Design review of the part built by this model. Coordinates are the model's own, in mm. Face numbers are marked on the shaded views. A direction names the side the tool comes from. Coordinates: 2 decimals unless noted, no trailing zeros. Loops run counter-clockwise (first coordinate to the right, second up) from the corner with the lowest first, then second, coordinate; pieces in that order, holes last. Notation, with made-up numbers: M 59,40.5 L 75,40.5 A19 ccw 75,48.5 Z; hole C 26,-13 d8. An arc over 180 degrees is marked long. Put each result on its own line as item: value. Start each with the question number.
(1) Take a section at C-C, the plane z = -11.5. Give the boundary of the cut face in (x, y), then the cut area to 3 significant figures.
(2) For the marked faces 1, 2, 3, 4 and 5, list the 3-axis set-ups (+Z, -Z, +X, -X, +Y, -Y) from which the entire face can be reached by the end or side of a thin tool; tool diameter is ignored.
(3) For probe 1 along Z at (x, y) = (36, 1.6); probe 2 along Y at (x, z) = (-22, -31.5), list the stretches that pass through material, from the lowest coordinate up. Write a range as [from, to].
(4) Take a section at B-B, the plane z = -36. Give the boundary of the cut face in (x, y).
(5) Clearance check with flat-ended pins moving along their axes: pin 1 (1 mm diameter, centred on x = -15.5, y = 11, fed in from +Z); pin 2 (5 mm diameter, centred on y = 10.5, z = -27, fed in from +X); pin 3 (2 mm diameter, centred on x = -1, y = 16.5, fed in from -Z). State where each tip first meets the part, or that it passes through.
(6) Take a section at D-D, the plane x = 26.5. Give the boundary of the cut face in (y, z), then the cut area to 3 significant figures.
(7) Take a section at A-A, the plane x = -36. Give the boundary of the cut face in (y, z).
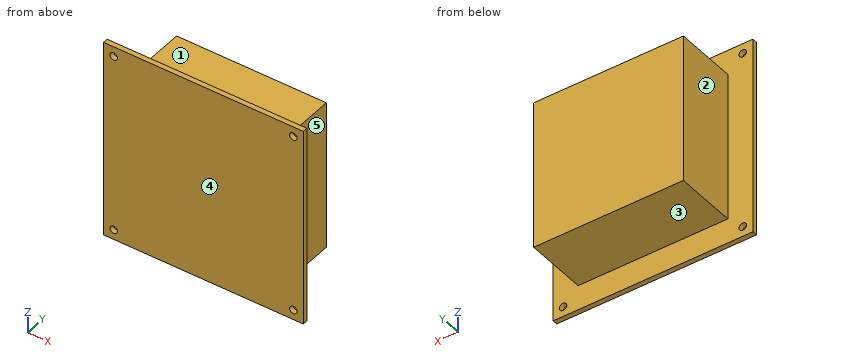
Autodesk Inventor part; units mm, degrees
ref_plane "YZ Plane" through (0, 0, 0) normal (1, 0, 0) x (0, 1, 0)
ref_plane "XZ Plane" through (0, 0, 0) normal (0, 1, 0) x (-1, 0, 0)
ref_plane "XY Plane" through (0, 0, 0) normal (0, 0, 1) x (1, 0, 0)
sketch "Esquisse1" plane through (0, 0, 0) normal (0, 1, 0) x (-1, 0, 0)
  line L0 (40, 40) -> (-40, 40)
  line L1 (-40, 40) -> (-40, -40)
  line L2 (-40, -40) -> (40, -40)
  line L3 (40, -40) -> (40, 40)
  point P0 (0, 0)
  dimension "d0" = 80
  dimension "d1" = 80
  dimension "d2" = 40
  dimension "d3" = 40
extrude "Extrusion1" add sketch "Esquisse1" along normal blind 2
sketch "Esquisse2" plane through (0, 2, 0) normal (0, 1, 0) x (1, 0, 0)
  line L0 (-36, -36) -> (36, -36) construction
  line L1 (36, -36) -> (36, 36) construction
  line L2 (36, 36) -> (-36, 36) construction
  line L3 (-36, 36) -> (-36, -36) construction
  circle A0 centre (-36, -36) radius 1.5
  circle A1 centre (-36, 36) radius 1.5
  circle A2 centre (36, 36) radius 1.5
  circle A3 centre (36, -36) radius 1.5
  point P0 (0, 0)
  dimension "d6" = 3
  dimension "d7" = 3
  dimension "d8" = 3
  dimension "d9" = 3
  dimension "d10" = 72
  dimension "d11" = 72
  dimension "d12" = 36
  dimension "d13" = 36
extrude "Extrusion2" cut sketch "Esquisse2" against normal through all
sketch "Esquisse3" plane through (0, 2, 0) normal (0, 1, 0) x (1, 0, 0)
  line L0 (-30, -30) -> (30, -30)
  line L1 (30, -30) -> (30, 30)
  line L2 (30, 30) -> (-30, 30)
  line L3 (-30, 30) -> (-30, -30)
  point P0 (0, 0)
  dimension "d16" = 60
  dimension "d17" = 60
  dimension "d18" = 30
  dimension "d19" = 30
extrude "Extrusion3" add sketch "Esquisse3" along normal blind 24.79
equation "\"d7\" = d6"
equation "\"d8\" = d6"
equation "\"d9\" = d6"
properties part number "rolling_base_board"
Computed values:
1. outline: M -40,0 L 40,0 L 40,2 L 30,2 L 30,26.79 L -30,26.79 L -30,2 L -40,2 Z
1. area: 1,650 mm^2
2. face 1: +Z, +X, -X, +Y
2. face 2: +Z, -Z, -X, +Y
2. face 3: -Z, +X, -X, +Y
2. face 4: +Z, -Z, +X, -X, -Y
2. face 5: +Z, -Z, +X, +Y
3. probe 1: z = [-40, -37.5], [-34.5, 34.5], [37.5, 40]
3. probe 2: y = [0, 2]
4. outline: M -40,0 L -37.5,0 L -37.5,2 L -40,2 Z; M -34.5,0 L 34.5,0 L 34.5,2 L -34.5,2 Z; M 37.5,0 L 40,0 L 40,2 L 37.5,2 Z
5. pin 1: stops at z = 30
5. pin 2: stops at x = 30
5. pin 3: stops at z = -30
6. outline: M 0,-40 L 2,-40 L 2,-30 L 26.79,-30 L 26.79,30 L 2,30 L 2,40 L 0,40 Z
6. area: 1,650 mm^2
7. outline: M 0,-40 L 2,-40 L 2,-37.5 L 0,-37.5 Z; M 0,-34.5 L 2,-34.5 L 2,34.5 L 0,34.5 Z; M 0,37.5 L 2,37.5 L 2,40 L 0,40 Z
